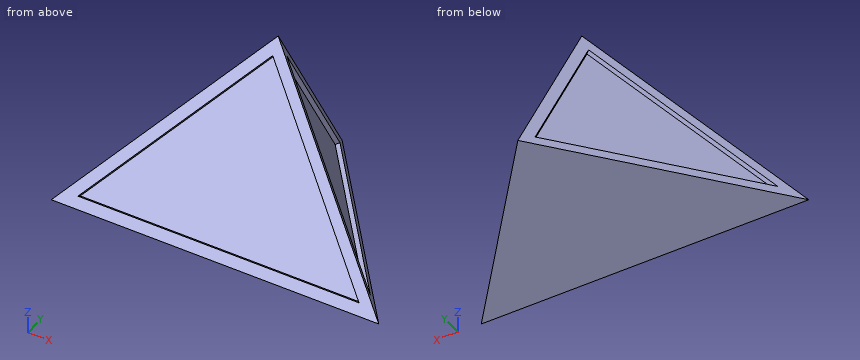
```python
from build123d import *

# Parameters (mm, degrees)
F7_DEPTH = 0.8128
F8_DEPTH = 0.8128
F9_DEPTH = 0.8128


with BuildPart() as f3:
    # F0 (on Top) → F3 section 0
    with BuildSketch(Plane.XY, mode=Mode.PRIVATE) as f3_s0:
        Polygon((-29.9980398268, -36.9558446109), (29.9980398268, -36.9558446109), (0, 0), align=None)
    loft([f3_s0.sketch, Vertex(-0.0778641552, -18.4707883745, 32.0170565822)])

    # F5 (on face) → F7 (cut)
    with BuildSketch(Plane(origin=(0, -27.7168834582, 16.0023501257), x_dir=(1, 0, 0), z_dir=(0, -0.8660254038, 0.5))):
        Polygon((-25.7607347469, -16.4560821702), (25.7468520606, -16.4560821702), (-0.0737889564, 15.2833462803), align=None)
    extrude(amount=-F7_DEPTH, mode=Mode.SUBTRACT)

    # F6 (on face) → F8 (cut)
    with BuildSketch(Plane(origin=(0, 0, 0), x_dir=(-0.5355684781, 0.8059841071, -0.252103202), z_dir=(0.729232256, 0.591937175, 0.3432647631))):
        Polygon((-41.7223640249, -9.5028096175), (-3.510395555, 1.1444631503), (-22.6090033778, 25.3135608223), align=None)
    extrude(amount=-F8_DEPTH, mode=Mode.SUBTRACT)

    # F4 (on face) → F9 (cut)
    with BuildSketch(Plane(origin=(0, 0, 0), x_dir=(-0.537220985, -0.805456085, 0.250268073), z_dir=(-0.7301171424, 0.5926554607, 0.3401300682))):
        Polygon((3.4951138194, 1.1430482538), (41.776044137, -9.426033441), (22.6281892536, 25.3299917255), align=None)
    extrude(amount=-F9_DEPTH, mode=Mode.SUBTRACT)


solid = f3.part
```
The model under review builds one solid part; all positions refer to its coordinate system, in mm. Round coordinates to 2 decimals unless told otherwise and drop trailing zeros. Loops run counter-clockwise (first coordinate to the right, second up) from the corner with the lowest first, then second, coordinate; pieces in that order, holes last. Notation, with made-up numbers: M 57.25,-9 L 80.25,-9 A22 cw 80.25,18 Z; hole C 8,26.5 d6. An arc over 180 degrees is marked long. Answer as a JSON object with one key per item and string values.
(1) Take a section at B-B on x = -13. Give the boundary of the cut face in (y, z), and give its area (3 significant figures).
Resolved:
{"outline": "M -36.96,0 L -16.02,0 L -17.11,1.91 L -18.32,1.63 L -26.2,15.36 L -25.36,16.28 L -26.45,18.19 L -28.06,15.41 L -27.36,15 L -35.24,1.34 L -35.94,1.75 Z", "area": "158 mm²"}
(2) Take a section at C-C on y = -23.5. Give the boundary of the cut face in (x, z), and give its area (3 significant figures).
Resolved:
{"outline": "M -19.08,0 L 19.08,0 L 18.17,1.92 L 17.19,1.64 L 8.54,20.02 L 9.91,19.46 L 8.1,23.31 L 5.5,23.31 L 6.64,21.68 L -6.76,21.68 L -5.62,23.31 L -8.22,23.31 L -10,19.49 L -8.62,20.05 L -17.2,1.63 L -18.19,1.91 Z", "area": "575 mm²"}
(3) Take a section at D-D on x = -19. Give the boundary of the cut face in (y, z), and give its area (3 significant figures).
Resolved:
{"outline": "M -36.96,0 L -23.41,0 L -24.5,1.91 L -25.72,1.63 L -29.91,8.94 L -29.06,9.85 L -30.16,11.77 L -31.77,8.99 L -31.06,8.58 L -35.24,1.34 L -35.94,1.75 Z", "area": "62.5 mm²"}
(4) Take a section at A-A on z = 24. Give the boundary of the cut face in (x, y), and give its area (3 significant figures).
Resolved:
{"outline": "M -7.57,-23.1 L -4.97,-23.1 L -4.59,-22.16 L 4.46,-22.16 L 4.85,-23.1 L 7.45,-23.1 L 5.65,-20.88 L 4.8,-21.2 L 0.75,-16.21 L 1.34,-15.57 L -0.06,-13.85 L -1.45,-15.56 L -0.86,-16.2 L -4.93,-21.22 L -5.78,-20.9 Z", "area": "49.1 mm²"}
(5) Clearance check with flat-ended pins moving along their axes: P1, Ø10, axis at x = 8.5, z = 23.5, coming from the +Y side; P2, Ø5, axis at y = -13, z = 27, coming from the +X side; P3, Ø8, axis at x = -17.5, z = 24, coming from the +Y side; P4, Ø10, axis at y = -24.5, z = 18, coming from the +X side. State where each tip first meets the part, or that it passes through.
Resolved:
{"P1": "y = -18.66", "P2": "x = 0.19", "P3": "through", "P4": "x = 16.05"}
(6) To check wall thickness, follow line 1 along Z through (x, y) = (-4, -22); line 2 along X through (y, z) = (-17.5, 29.5); line 3 along Z through (x, y) = (2, -7). State the ranges of each line that lie inside material, in increasing order.
Resolved:
{"line 1": "0 to 24.28, 24.75 to 25.9", "line 2": "-0.46 to 0.32", "line 3": "0 to 5.45"}
